Work out the finished part from the listing and answer in its coordinate system (mm). A direction names the side the tool comes from. Give positions to 0.01 mm unless a question says otherwise; leave off trailing zeros. Loops run counter-clockwise (first coordinate to the right, second up) from the corner with the lowest first, then second, coordinate; pieces in that order, holes last. Notation, with made-up numbers: M -27.5,-30 L -11.5,-30 A25 ccw -11.5,-3 Z; hole C 19.25,6.5 d2. An arc over 180 degrees is marked long. Use a Markdown table: item, result.
```python
from build123d import *

# Parameters (mm, degrees)
SKETCH1_R           = 5.75
SKETCH1_R_2         = 2
BOSS_EXTRUDE1_DEPTH = 340
SKETCH33_R          = 16.5
BOSS_EXTRUDE2_DEPTH = 7
BOSS_EXTRUDE5_START = -10
SKETCH1_4_R         = 5.75
SKETCH1_4_R_2       = 2
BOSS_EXTRUDE5_DEPTH = 10
SKETCH38_R          = 2.125
CUT_EXTRUDE1_DEPTH  = 8
BOSS_EXTRUDE6_START = 8
BOSS_EXTRUDE6_DEPTH = 8
SKETCH40_R          = 1.5
CUT_EXTRUDE2_DEPTH  = 10


with BuildPart() as part:
    # Sketch1 → Boss-Extrude1 (new body)
    # profile 1 of 2: a face of its own
    with BuildSketch(Plane(origin=(0, 0, 0), x_dir=(1, 0, 0), z_dir=(0, 1, 0))):
        with Locations(Location((0, 0, 0), (0, 0, 270))):
            Circle(SKETCH1_R)
        Circle(SKETCH1_R_2, mode=Mode.SUBTRACT)
    # profile 2 of 2: a face of its own
    with BuildSketch(Plane(origin=(0, 0, 0), x_dir=(1, 0, 0), z_dir=(0, 1, 0))):
        Circle(SKETCH1_R_2)
    extrude(amount=BOSS_EXTRUDE1_DEPTH)

    # Sketch33 → Boss-Extrude2 (add)
    with BuildSketch(Plane.XZ):
        with Locations(Location((0, 0, 0), (0, 0, 270))):
            Circle(SKETCH33_R)
    extrude(amount=-BOSS_EXTRUDE2_DEPTH)

    # Sketch1<4> → Boss-Extrude5 (add)
    # profile 1 of 2: a face of its own
    with BuildSketch(Plane(origin=(0, 0, 0), x_dir=(1, 0, 0), z_dir=(0, 1, 0)).offset(BOSS_EXTRUDE5_START)):
        with Locations(Location((0, 0, 0), (0, 0, 90))):
            Circle(SKETCH1_4_R)
        Circle(SKETCH1_4_R_2, mode=Mode.SUBTRACT)
    # profile 2 of 2: a face of its own
    with BuildSketch(Plane(origin=(0, 0, 0), x_dir=(1, 0, 0), z_dir=(0, 1, 0)).offset(BOSS_EXTRUDE5_START)):
        Circle(SKETCH1_4_R_2)
    extrude(amount=BOSS_EXTRUDE5_DEPTH)

    # Sketch38 → Cut-Extrude1 (cut)
    with BuildSketch(Plane.XZ.offset(10)):
        with Locations(Location((0, 0, 0), (0, 0, 270))):
            Circle(SKETCH38_R)
    extrude(amount=-CUT_EXTRUDE1_DEPTH, mode=Mode.SUBTRACT)

    # Sketch39 → Boss-Extrude6 (add)
    with BuildSketch(Plane.XZ.offset(2).offset(BOSS_EXTRUDE6_START)):
        with BuildLine():
            ThreePointArc((1.398436627, 1.6), (0, 2.125), (-1.398436627, 1.6))
            Line((-1.398436627, 1.6), (1.398436627, 1.6))
        make_face()
    extrude(amount=-BOSS_EXTRUDE6_DEPTH)

    # Sketch40 → Cut-Extrude2 (cut)
    with BuildSketch(Plane(origin=(0, 340, 0), x_dir=(1, 0, 0), z_dir=(0, 1, 0))):
        with Locations(Location((0, 0, 0), (0, 0, 270))):
            Circle(SKETCH40_R)
    extrude(amount=-CUT_EXTRUDE2_DEPTH, mode=Mode.SUBTRACT)


solid = part.part
```
(1) Which of the six approach directions +Z, -Z, +X, -X, +Y, -Y give full straight-line access (tool end or side, diameter ignored) to faces 1 (the flat face through (-0.1, -10, -2.5)), 2 (the cylindrical face through (-4.85, -5.07, -3.09)), 3 (the cylindrical face through (4.85, 171.17, 3.09))?
Entries:
| item | result |
|---|---|
| face 1 | +Z, -Z, +X, -X, -Y |
| face 2 | -Y |
| face 3 | +Y |
(2) A cutting plane is placed at B-B (x = 13.5). Write down the section's boundary in (y, z).
Entries:
| item | result |
|---|---|
| outline | M 0,-9.49 L 7,-9.49 L 7,9.49 L 0,9.49 Z |
(3) A cutting plane is placed at A-A (y = 161.5). Write down the section's boundary in (x, z).
Entries:
| item | result |
|---|---|
| outline | C 0,0 d11.5 |
(4) A cutting plane is placed at C-C (z = 12). Write down the section's boundary in (x, y).
Entries:
| item | result |
|---|---|
| outline | M -11.32,0 L 11.32,0 L 11.32,7 L -11.32,7 Z |
(5) Given P1, Ø2, axis at y = 52, z = 3.5, coming from the +X side; P2, Ø5, axis at y = 291, z = 0.5, coming from the -X side; P3, Ø2.5, axis at x = 0, z = 0, coming from the -Y side; P4, Ø16.5, axis at x = -0.5, z = -7, coming from the -Y side, each flat-ended and moving along its own axis, determine where each tip first touches the part or whether it passes through.
Entries:
| item | result |
|---|---|
| P1 | stops at x = 5.18 |
| P2 | stops at x = -5.75 |
| P3 | stops at y = -2 |
| P4 | stops at y = -10 |
(6) Consider probe 1 along X at (y, z) = (337.5, 0); probe 2 along Y at (x, z) = (9, -11.5); probe 3 along X at (y, z) = (-5.25, 0) (3 decimals). Determine where each line is inside the solid, lowest interval first. Write a range as [from, to].
Entries:
| item | result |
|---|---|
| probe 1 | x = [-5.75, -1.5], [1.5, 5.75] |
| probe 2 | y = [0, 7] |
| probe 3 | x = [-5.75, -2.125], [2.125, 5.75] |
